The model under review builds one solid part; all positions refer to its coordinate system, in mm. Round coordinates to 2 decimals unless told otherwise and drop trailing zeros. Order: outer loops, then holes, each group sorted by start corner. A loop starts at its lowest first (then second) coordinate and runs counter-clockwise, first axis right, second up. Notation, with made-up numbers: M 54.25,70 L 92.25,70 A35 ccw 92.25,107 Z; hole C 63,13 d3. An arc over 180 degrees is marked long. Answer as a JSON object with one key per item and string values. Group by question number.
1) To check wall thickness, follow line 1 (X direction, y = 11.5, z = 6); line 2 (X direction, y = 13.5, z = 0); line 3 (Y direction, x = 11, z = -11). State the ranges of each line that lie inside material, in increasing order.
2) Insertion check: pin 1 Ø8 at (y, z) = (13, 25) entering from -X; pin 2 Ø2 at (y, z) = (13.5, -23) entering from +X. Each pin has a flat end and moves straight along its axis. Give the tip position at first contact, or say it passes through.
3) Consider section A-A, the plane z = -14. Write out the cut boundary in (x, y), then the cut area to 3 significant figures.
```python
from build123d import *

# Parameters (mm, degrees)
F0_W     = 25.4
F0_H     = 63.5
F1_DEPTH = 17.78
F2_R     = 6.35
F3_R     = 5.08


with BuildPart() as f1:
    # F0 (on Front) → F1 (new body, symmetric)
    with BuildSketch(Plane.XZ):
        Rectangle(F0_W, F0_H)
    extrude(amount=F1_DEPTH, both=True)

    # F2
    f2_edges = [f1.edges().sort_by_distance(p)[0] for p in [
        (-12.7, -17.78, 0),
        (-12.7, 17.78, 0),
        (12.7, 17.78, 0),
        (12.7, -17.78, 0),
    ]]
    fillet(f2_edges, radius=F2_R)

    # F3
    f3_edges = [f1.edges().sort_by_distance(p)[0] for p in [
        (0, 17.78, -31.75),
        (-10.840128, 15.920128, -31.75),
        (10.840128, 15.920128, -31.75),
        (-12.7, 0, -31.75),
        (12.7, 0, -31.75),
        (-10.840128, -15.920128, -31.75),
        (10.840128, -15.920128, -31.75),
        (0, -17.78, -31.75),
    ]]
    fillet(f3_edges, radius=F3_R)


solid = f1.part
```
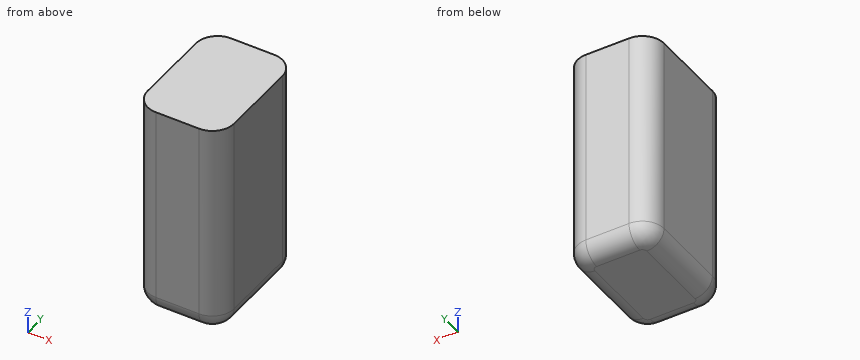
Results list:
{
 "1": {"line 1": "-12.7 to 12.7", "line 2": "-12.35 to 12.35", "line 3": "-15.75 to 15.75"},
 "2": {"pin 1": "x = -12.7", "pin 2": "x = 12.61"},
 "3": {"outline": "M -12.7,-11.43 A6.35 ccw -6.35,-17.78 L 6.35,-17.78 A6.35 ccw 12.7,-11.43 L 12.7,11.43 A6.35 ccw 6.35,17.78 L -6.35,17.78 A6.35 ccw -12.7,11.43 Z", "area": "869 mm^2"}
}
